Work out the finished part from the listing and answer in its coordinate system (mm). Face numbers are marked on the shaded views. A direction names the side the tool comes from. Round coordinates to 2 decimals unless told otherwise and drop trailing zeros. Order: outer loops, then holes, each group sorted by start corner. A loop starts at its lowest first (then second) coordinate and runs counter-clockwise, first axis right, second up. Notation, with made-up numbers: M -11.75,-37.5 L 11.25,-37.5 A17 ccw 11.25,-33.5 Z; hole C 18.5,70.25 d11. An arc over 180 degrees is marked long. Answer as a JSON object with one key per item and string values. Group by question number.
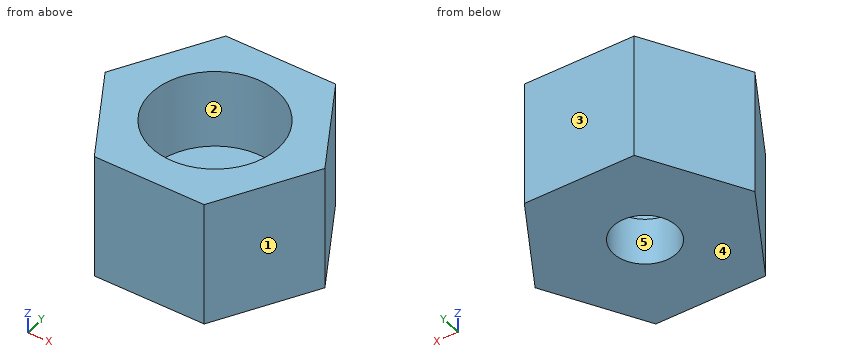
from build123d import *

# Parameters (mm, degrees)
SKETCH1_R           = 2
BOSS_EXTRUDE1_DEPTH = 4
SKETCH2_R           = 4
CUT_EXTRUDE1_DEPTH  = 5


with BuildPart() as part:
    # Sketch1 → Boss-Extrude1 (new, symmetric)
    with BuildSketch(Plane.XY):
        Polygon((6.92820323, 0), (3.464101615, 6), (-3.464101615, 6), (-6.92820323, 0), (-3.464101615, -6), (3.464101615, -6), align=None)
        Circle(SKETCH1_R, mode=Mode.SUBTRACT)
    extrude(amount=BOSS_EXTRUDE1_DEPTH, both=True)

    # Sketch2 → Cut-Extrude1 (cut)
    with BuildSketch(Plane.XY.offset(4)):
        Circle(SKETCH2_R)
    extrude(amount=-CUT_EXTRUDE1_DEPTH, mode=Mode.SUBTRACT)


solid = part.part
Item 1: Find section C-C (z = 0.25). Give the vertices of the cut face in (x, y), and give its area (3 significant figures).
Item 2: Find section B-B (y = -1). Give the vertices of the cut face in (x, z).
Item 3: Find section A-A (x = 0). Give the vertices of the cut face in (y, z), and give its area (3 significant figures).
Item 4: The mould has two halves that part along Y. Classify the marked faces 3, 4 and 5: +Y half, -Y half, draft (parallel to the pull), parting line (faces both ways), or undercut.
Item 5: Consider L1, parallel to Y at x = 0, z = -2.5; L2, parallel to Y at x = 0, z = 0.5; L3, parallel to Z at x = 0.5, y = -2. Determine where each line is inside the solid, lowest interval first.
Item 6: Find section D-D (x = 2.25). Give the vertices of the cut face in (y, z).
Item 7: This flat-tipped pin is pushed along its axis until it touches: pin 1 (2 mm diameter, centred on y = 2, z = 3, fed in from -X). Where does it stop, or does it pass through?
Item 8: A tool of negligible diameter and unlimited length cuts with its end or side. For the marked faces 1 and 2, from which of +Z, -Z, +X, -X, +Y, -Y can it reach the whole face along a straight path? Write none if from no direction.
Responses:
{
 "1": {"outline": "M -6.93,0 L -3.46,-6 L 3.46,-6 L 6.93,0 L 3.46,6 L -3.46,6 Z; hole C 0,0 d8", "area": "74.4 mm^2"},
 "2": {"outline": "M -6.35,-4 L -1.73,-4 L -1.73,-1 L -3.87,-1 L -3.87,4 L -6.35,4 Z; M 1.73,-4 L 6.35,-4 L 6.35,4 L 3.87,4 L 3.87,-1 L 1.73,-1 Z"},
 "3": {"outline": "M -6,-4 L -2,-4 L -2,-1 L -4,-1 L -4,4 L -6,4 Z; M 2,-4 L 6,-4 L 6,4 L 4,4 L 4,-1 L 2,-1 Z", "area": "44.0 mm^2"},
 "4": {"face 3": "+Y half", "face 4": "draft", "face 5": "undercut"},
 "5": {"L1": "y = -6 to -2, 2 to 6", "L2": "y = -6 to -4, 4 to 6", "L3": "z = -4 to -1"},
 "6": {"outline": "M -6,-4 L 6,-4 L 6,4 L 3.31,4 L 3.31,-1 L -3.31,-1 L -3.31,4 L -6,4 Z"},
 "7": {"pin 1": "stops at x = -6.35"},
 "8": {"face 1": "+Z, -Z, +X, -Y", "face 2": "+Z"}
}
